Work out the finished part from the listing and answer in its coordinate system (mm). A direction names the side the tool comes from. Give positions to 0.01 mm unless a question says otherwise; leave off trailing zeros. Order: outer loops, then holes, each group sorted by start corner. A loop starts at its lowest first (then second) coordinate and runs counter-clockwise, first axis right, second up.
```python
from build123d import *

# Parameters (mm, degrees)
SKETCH1_R              = 3.5
BOSS_EXTRUDE1_DEPTH    = 13
F_25_0MM_DOWEL_HOLE1_D = 35


with BuildPart() as part:
    # Sketch1 → Boss-Extrude1 (new body)
    with BuildSketch(Plane.XY):
        Polygon((-103.143983002, 33.195876289), (-53.143983002, 33.195876289), (-53.143983002, 20), (16.856016998, 20), (16.856016998, 33.195876289), (66.856016998, 33.195876289), (66.856016998, 20), (126.856016998, 20), (126.856016998, 33.195876289), (176.856016998, 33.195876289), (176.856016998, 20), (316.856016998, 20), (316.856016998, -20), (176.856016998, -20), (176.856016998, -33.195876289), (126.856016998, -33.195876289), (126.856016998, -20), (66.856016998, -20), (66.856016998, -33.195876289), (16.856016998, -33.195876289), (16.856016998, -20), (-53.143983002, -20), (-53.143983002, -33.195876289), (-103.143983002, -33.195876289), (-103.143983002, -20), (-163.143983002, -20), (-163.143983002, 20), (-103.143983002, 20), align=None)
        with Locations(Location((-74.643983002, 25, 0), (0, 0, 180))):
            Circle(SKETCH1_R, mode=Mode.SUBTRACT)
        with Locations(Location((155.356016998, 25, 0), (0, 0, 180))):
            Circle(SKETCH1_R, mode=Mode.SUBTRACT)
        with Locations(Location((155.356016998, -25, 0), (0, 0, 180))):
            Circle(SKETCH1_R, mode=Mode.SUBTRACT)
        with Locations(Location((-74.643983002, -25, 0), (0, 0, 180))):
            Circle(SKETCH1_R, mode=Mode.SUBTRACT)
    extrude(amount=BOSS_EXTRUDE1_DEPTH)

    # Ø25.0mm Dowel Hole1 (through all)
    with Locations(Plane(origin=(41.856016998, 0, 13), x_dir=(1, 0, 0), z_dir=(0, 0, 1))):
        with Locations((0, 0)):
            Hole(F_25_0MM_DOWEL_HOLE1_D / 2)


solid = part.part
```
1. The part is cut by section A-A (y = 0). Write down the section's boundary in (x, z).
Findings below:
outline: (-163.14, 0) - (24.36, 0) - (24.36, 13) - (-163.14, 13) - close; (59.36, 0) - (316.86, 0) - (316.86, 13) - (59.36, 13) - close
2. Given P1, Ø4, axis at y = 26.5, z = 5.5, coming from the -X side; P2, Ø6.5, axis at y = 25, z = 6.5, coming from the +X side; P3, Ø4, axis at x = 95, z = 8.5, coming from the +Y side, each flat-ended and moving along its own axis, determine where each tip first touches the part or whether it passes through.
Findings below:
P1: stops at x = -103.14
P2: stops at x = 176.86
P3: stops at y = 20
3. The mould has two halves that part along Y. Classify faces 6 (the face through (-53.144, 27, 6)), 7 (the face through (55.74, -10.65, 6.41)), 8 (the face through (-18, -20, 6)), 9 (the face through (42, 33.196, 6)): pulls with the +Y half, pulls with the -Y half, needs draft (parallel to the pull), parting line crosses it, or undercut.
Findings below:
face 6: needs draft
face 7: undercut
face 8: pulls with the -Y half
face 9: pulls with the +Y half
4. Straight lines are drawn through the part: probe 1 along X at (y, z) = (-25, 4); probe 2 along Y at (x, z) = (100.5, 8.25); probe 3 along X at (y, z) = (27, 10.25). For each, find the intervals that lie inside material, in ascending order.
Findings below:
probe 1: x = -103.14 to -78.14, -71.14 to -53.14, 16.86 to 66.86, 126.86 to 151.86, 158.86 to 176.86
probe 2: y = -20 to 20
probe 3: x = -103.14 to -77.52, -71.77 to -53.14, 16.86 to 66.86, 126.86 to 152.48, 158.23 to 176.86
5. The part is cut by section C-C (x = 29). Write down the section's boundary in (y, z).
Findings below:
outline: (-33.2, 0) - (-11.87, 0) - (-11.87, 13) - (-33.2, 13) - close; (11.87, 0) - (33.2, 0) - (33.2, 13) - (11.87, 13) - close
6. Which of the six approach directions +Z, -Z, +X, -X, +Y, -Y give full straight-line access (tool end or side, diameter ignored) to faces 1 (the face through (-133, -20, 6)), 2 (the face through (246, 20, 6)), 3 (the face through (66.856, 27, 6)), 4 (the face through (66.856, -27, 6)), 5 (the face through (248, -20, 6))?
Findings below:
face 1: +Z, -Z, -X, -Y
face 2: +Z, -Z, +X, +Y
face 3: +Z, -Z, +Y
face 4: +Z, -Z, -Y
face 5: +Z, -Z, +X, -Y
7. The part is cut by section B-B (z = 4). State how many separate pieces and enclosed holes the cut face has, then the cut area to 3 significant figures.
Findings below:
separate pieces: 1
enclosed holes: 5
area: 22,000 mm2
